Autodesk Inventor part; units mm, degrees
ref_plane "Work Plane1" through (29, 0, 0) normal (0, -1, 0) x (1, 0, 0)
ref_plane "YZ Plane" through (0, 0, 0) normal (1, 0, 0) x (0, 1, 0)
ref_plane "XZ Plane" through (0, 0, 0) normal (0, 1, 0) x (-1, 0, 0)
sketch "Sketch1" plane through (0, 0, 0) normal (0, 0, 1) x (1, 0, 0)
  line L0 (0.0567, 0) -> (12, 0)
  line L1 (12, 0) -> (12, 1.5)
  line L2 (12, 1.5) -> (1, 1.5)
  line L3 (1, 1.5) -> (0.6932, 1.5)
  line L4 (0.6932, 1.5) -> (0, 1.5)
  line L5 (0, 1.5) -> (0, 2.85)
  line L6 (0, 2.85) -> (-1.65, 2.85)
  line L7 (-1.65, 2.85) -> (-1.65, 1.1547)
  line L8 (-1.65, 1.1547) -> (-0.61, 1.1547)
  line L9 (-0.61, 1.1547) -> (0.0567, 0)
  line L10 (-4.38, 0) -> (14.73, 0)
  line L11 (0, -0.57) -> (0, 3.42)
  line L12 (1, 1.5) -> (0, 1.5) construction
  dimension "d1" = 11
  dimension "d2" = 0.3068
  dimension "d3" = 1.65
  dimension "d4" = 1.04
  dimension "d5" = 60
  dimension "d6" = 3
  dimension "d7" = 3
  dimension "d8" = 2.3094
  dimension "d9" = 5.7
  dimension "d26" = 12
revolve "Body" add sketch "Sketch1" angle 360 about axis through (0.0567, 0, 0) along (1, 0, 0) contours L9 L11 L4 L3 L2 L1 L0 | L9 L8 L7 L6 L5 L11
sketch "Sketch2" plane through (-1.65, 0, 0) normal (-1, 0, 0) x (0, 0, 1)
  circle A0 centre (0, 0) radius 1.1547
  line L0 (0, -3.99) -> (0, 3.99)
  line L1 (-3.99, 0) -> (3.99, 0)
  line L2 (1.1547, 0) -> (0.5774, -1)
  line L3 (0.5774, -1) -> (-0.5774, -1)
  line L4 (-0.5774, -1) -> (-1.1547, 0)
  line L5 (-1.1547, 0) -> (-0.5774, 1)
  line L6 (-0.5774, 1) -> (0.5774, 1)
  line L7 (0.5774, 1) -> (1.1547, 0)
extrude "Slot" add sketch "Sketch2" against normal up to next contours L7 A0 | A0 L2 | L6 L0 A0 | A0 L0 L3 | L0 L6 A0 | A0 L3 L0 | L4 A0 | A0 L5
fillet "Fillet1" radius 1.45 1 edges at (-1.65, -2.85, 0)
thread "Thread"
chamfer "Chamfer1" distance 0.3067 distance2 0.3067 1 edges at (12, -1.5, 0) measured on face at (12, -0.6587, -0.1791)
ref_plane "Work Plane1" through (29, 0, 0) normal (0, -1, 0) x (1, 0, 0)
fillet "Fillet2" radius 0.1 1 edges at (0, -1.5, 0)
equation "\"d1\" = GEL"
equation "\"d3\" = KOH"
equation "\"d4\" = INTI"
equation "\"d6\" = GD"
equation "\"d7\" = BDM"
equation "\"d8\" = 1.1547 * SW"
equation "\"d9\" = KOD"
equation "\"d26\" = NLG"
equation "\"d30\" = R"
equation "\"d17\" = RR"
equation "\"d13\" = GEL"
equation "\"d15\" = -0.5 * SPD + 0.5 * GD"
equation "\"d16\" = GUL"
equation "\"GD\" = 3"
equation "\"NLG\" = 12"
equation "\"GEL\" = 11"
equation "\"KOD\" = 5.7"
equation "\"KOH\" = 1.65"
equation "\"INTI\" = 1.04"
equation "\"GAL\" = 0.61345 * PTC"
equation "\"GUL\" = 0.61345 * PTC"
equation "\"BDM\" = 3"
equation "\"SW\" = 2"
equation "\"RR\" = 1.45"
equation "\"SPD\" = NND - 1.2269 * PTC"
equation "\"R\" = 0.1"
equation "\"TOA\" = 30deg"
equation "\"GD1\" = THREADDIA - 1.2269 * PTC"
equation "\"THREADDIA\" = 3"
equation "\"PTC\" = 0.5"
equation "\"NND\" = 3"
equation "\"KOH1\" = 0.2"
equation "\"E0\" = 2.31"
properties part number "Screw GB/T 70.2 M3 X 12" material "Steel, Mild"
Geometry: final body of the model. Coordinates: model frame, mm. A direction names the side the tool comes from. Coordinates: 2 decimals unless noted, no trailing zeros. Order: outer loops, then holes, each group sorted by start corner. A loop starts at its lowest first (then second) coordinate and runs counter-clockwise, first axis right, second up. Notation, with made-up numbers: (69, 59) - (94, 59) arc R16 ccw to (94, 68) - close; hole circle Ø6 at (51.5, 28). An arc over 180 degrees is marked (long way). Use one line per item in the form item = value.
1) Pin query (flat end, axial travel): pin 1 (2 mm diameter, centred on x = 8, z = 0.5, fed in from +Y); pin 2 (1.5 mm diameter, centred on x = 3.5, y = 2, fed in from -Z); pin 3 (1.5 mm diameter, centred on x = 6, y = 1.5, fed in from -Z). Return the tip coordinate at first contact, or that it passes through.
Solutions:
pin_1 = 1.5
pin_2 = -0.83
pin_3 = -1.3
2) Ray query, L1, parallel to Z at x = -1, y = -0.65; L2, parallel to X at y = 0.7, z = 1.5; L3, parallel to Z at x = 4.5, y = 0.5. Return the intervals inside material, ascending.
Solutions:
L1 = -2.53 to -0.78, 0.78 to 2.53
L2 = -1.63 to 0
L3 = -1.41 to 1.41
3) Section A-A (x = 9.75). Return loops of the section in (y, z).
Solutions:
outline = circle Ø3 at (0, 0)
4) Set-up query: faces 4 (the face through (-1, -1, 0)), 5 (the face through (12, 0, 0)). Return all of +Z, -Z, +X, -X, +Y, -Y with unobstructed straight access to the full face (end or side cutting, diameter ignored); none if empty.
Solutions:
face_4 = -X
face_5 = +Z, -Z, +X, +Y, -Y
5) Mould query, pull axis Y, two halves, no side actions, for faces 1 (the face through (-1, 1, 0)), 2 (the face through (5.82, -1.5, -0.07)), 3 (the face through (0, 0, -2)). Classes: +Y half, -Y half, draft (parallel to the pull), parting line (faces both ways), or undercut.
Solutions:
face_1 = undercut
face_2 = parting line
face_3 = draft
